Design review of the part built by this model. Coordinates are the model's own, in mm. A direction names the side the tool comes from. Coordinates: 2 decimals unless noted, no trailing zeros. Order: outer loops, then holes, each group sorted by start corner. A loop starts at its lowest first (then second) coordinate and runs counter-clockwise, first axis right, second up.
from build123d import *

# Parameters (mm, degrees)
F1_DEPTH = 5


with BuildPart() as f1:
    # F0 (on Top) → F1 (new body)
    with BuildSketch(Plane.XY):
        Polygon((3, 75), (0, 75), (0, -75), (3, -75), (3, -25.685898), (3, -24.314102), (3, -21.685898), (3, -20.314102), (3, -17.685898), (3, -16.314102), (3, -13.685898), (3, -12.314102), (3, -9.685898), (3, -8.314102), (3, -5.685898), (3, -4.314102), (3, -1.685898), (3, -0.314102), (3, 2.314102), (3, 3.685898), (3, 6.314102), (3, 7.685898), (3, 10.314102), (3, 11.685898), (3, 14.314102), (3, 15.685898), (3, 18.314102), (3, 19.685898), (3, 22.314102), (3, 23.685898), (3, 26.314102), (3, 27.685898), align=None)
        with BuildLine():
            ThreePointArc((5, 27.15), (4.035276, 27.549602), (3, 27.685898))
            Line((3, 27.685898), (3, 26.314102))
            ThreePointArc((3, 26.314102), (4.035276, 26.450398), (5, 26.85))
            Line((5, 26.85), (5, 27))
            Line((5, 27), (5, 27.15))
        make_face()
        with BuildLine():
            Line((3, -24.314102), (3, -25.685898))
            ThreePointArc((3, -25.685898), (4.035276, -25.549602), (5, -25.15))
            Line((5, -25.15), (5, -25))
            Line((5, -25), (5, -24.85))
            ThreePointArc((5, -24.85), (4.035276, -24.450398), (3, -24.314102))
        make_face()
        with BuildLine():
            ThreePointArc((5, 23.15), (4.035276, 23.549602), (3, 23.685898))
            Line((3, 23.685898), (3, 22.314102))
            ThreePointArc((3, 22.314102), (4.035276, 22.450398), (5, 22.85))
            Line((5, 22.85), (5, 23))
            Line((5, 23), (5, 23.15))
        make_face()
        with BuildLine():
            Line((3, -20.314102), (3, -21.685898))
            ThreePointArc((3, -21.685898), (4.035276, -21.549602), (5, -21.15))
            Line((5, -21.15), (5, -21))
            Line((5, -21), (5, -20.85))
            ThreePointArc((5, -20.85), (4.035276, -20.450398), (3, -20.314102))
        make_face()
        with BuildLine():
            ThreePointArc((5, 19.15), (4.035276, 19.549602), (3, 19.685898))
            Line((3, 19.685898), (3, 18.314102))
            ThreePointArc((3, 18.314102), (4.035276, 18.450398), (5, 18.85))
            Line((5, 18.85), (5, 19))
            Line((5, 19), (5, 19.15))
        make_face()
        with BuildLine():
            Line((3, -16.314102), (3, -17.685898))
            ThreePointArc((3, -17.685898), (4.035276, -17.549602), (5, -17.15))
            Line((5, -17.15), (5, -17))
            Line((5, -17), (5, -16.85))
            ThreePointArc((5, -16.85), (4.035276, -16.450398), (3, -16.314102))
        make_face()
        with BuildLine():
            ThreePointArc((5, 15.15), (4.035276, 15.549602), (3, 15.685898))
            Line((3, 15.685898), (3, 14.314102))
            ThreePointArc((3, 14.314102), (4.035276, 14.450398), (5, 14.85))
            Line((5, 14.85), (5, 15))
            Line((5, 15), (5, 15.15))
        make_face()
        with BuildLine():
            Line((3, -12.314102), (3, -13.685898))
            ThreePointArc((3, -13.685898), (4.035276, -13.549602), (5, -13.15))
            Line((5, -13.15), (5, -13))
            Line((5, -13), (5, -12.85))
            ThreePointArc((5, -12.85), (4.035276, -12.450398), (3, -12.314102))
        make_face()
        with BuildLine():
            ThreePointArc((5, 11.15), (4.035276, 11.549602), (3, 11.685898))
            Line((3, 11.685898), (3, 10.314102))
            ThreePointArc((3, 10.314102), (4.035276, 10.450398), (5, 10.85))
            Line((5, 10.85), (5, 11))
            Line((5, 11), (5, 11.15))
        make_face()
        with BuildLine():
            Line((3, -8.314102), (3, -9.685898))
            ThreePointArc((3, -9.685898), (4.035276, -9.549602), (5, -9.15))
            Line((5, -9.15), (5, -9))
            Line((5, -9), (5, -8.85))
            ThreePointArc((5, -8.85), (4.035276, -8.450398), (3, -8.314102))
        make_face()
        with BuildLine():
            ThreePointArc((5, 7.15), (4.035276, 7.549602), (3, 7.685898))
            Line((3, 7.685898), (3, 6.314102))
            ThreePointArc((3, 6.314102), (4.035276, 6.450398), (5, 6.85))
            Line((5, 6.85), (5, 7))
            Line((5, 7), (5, 7.15))
        make_face()
        with BuildLine():
            Line((3, -4.314102), (3, -5.685898))
            ThreePointArc((3, -5.685898), (4.035276, -5.549602), (5, -5.15))
            Line((5, -5.15), (5, -5))
            Line((5, -5), (5, -4.85))
            ThreePointArc((5, -4.85), (4.035276, -4.450398), (3, -4.314102))
        make_face()
        with BuildLine():
            ThreePointArc((5, 3.15), (4.035276, 3.549602), (3, 3.685898))
            Line((3, 3.685898), (3, 2.314102))
            ThreePointArc((3, 2.314102), (4.035276, 2.450398), (5, 2.85))
            Line((5, 2.85), (5, 3))
            Line((5, 3), (5, 3.15))
        make_face()
        with BuildLine():
            Line((3, -0.314102), (3, -1.685898))
            ThreePointArc((3, -1.685898), (4.035276, -1.549602), (5, -1.15))
            Line((5, -1.15), (5, -1))
            Line((5, -1), (5, -0.85))
            ThreePointArc((5, -0.85), (4.035276, -0.450398), (3, -0.314102))
        make_face()
    extrude(amount=F1_DEPTH)

    # F2: F1 across face


with BuildPart() as f1_1:
    add(f1.part)
    add(f1.part.mirror(Plane(origin=(0, 0, 2.5), x_dir=(0, -1, 0), z_dir=(-1, 0, 0))))


solid = f1_1.part
1. Insertion check: pin 1 (0.8 mm diameter, centred on y = -19.5, z = 3, fed in from +X); pin 2 (1.3 mm diameter, centred on y = 21.5, z = 3.5, fed in from -X); pin 3 (6 mm diameter, centred on x = 2, y = 57.5, fed in from -Z). Each pin has a flat end and moves straight along its axis. Give the tip position at first contact, or say it passes through.
2. Add section A-A (y = -52). Give the boundary of the cut face in (x, z).
3. Mouldability with a two-part tool opening along Y and no side actions: class faces 1 (the flat face through (0, -75, 2)), 2 (the flat face through (3, 21, 2)), 3 (the flat face through (-3, 13, 2)), 4 (the flat face through (0, 1, 0)) as pulls with the +Y half, pulls with the -Y half, needs draft (parallel to the pull), parting line crosses it, or undercut.
4. To check wall thickness, follow line 1 (X direction, y = 34, z = 2.6). State the ranges of the line that lie inside material, in increasing order.
5. For faces 5 (the flat face through (-3, -23, 2)), 6 (the flat face through (-3, 51, 2)), 7 (the flat face through (3, -15, 2)), list the 3-axis set-ups (+Z, -Z, +X, -X, +Y, -Y) from which the entire face can be reached by the end or side of a thin tool; tool diameter is ignored.
Solution:
1. pin 1: stops at x = 3
1. pin 2: stops at x = -3
1. pin 3: stops at z = 0
2. outline: (-3, 0) - (3, 0) - (3, 5) - (-3, 5) - close
3. face 1: pulls with the -Y half
3. face 2: undercut
3. face 3: undercut
3. face 4: needs draft
4. line 1: x = -3 to 3
5. face 5: +Z, -Z, -X
5. face 6: +Z, -Z, -X, +Y
5. face 7: +Z, -Z, +X
